Design review of the part built by this model. Coordinates are the model's own, in mm. A direction names the side the tool comes from. Coordinates: 2 decimals unless noted, no trailing zeros. Order: outer loops, then holes, each group sorted by start corner. A loop starts at its lowest first (then second) coordinate and runs counter-clockwise, first axis right, second up. Notation, with made-up numbers: M 17,72 L 55,72 A17 ccw 55,82 Z; hole C 4,35.5 d10. An arc over 180 degrees is marked long. Answer in a Markdown table with one row per item.
from build123d import *

# Parameters (mm, degrees)
BOSS_EXTRUDE1_DEPTH = 40
CUT_EXTRUDE1_DEPTH  = 10


with BuildPart() as part:
    # Sketch1 → Boss-Extrude1 (new body)
    with BuildSketch(Plane.XY):
        Polygon((0, 0), (-7.54, -7.54), (-34.44, -7.54), (-34.44, -2.54), (-9.611067812, -2.54), (0, 7.071067812), (9.611067812, -2.54), (34.44, -2.54), (34.44, -7.54), (7.54, -7.54), align=None)
    extrude(amount=BOSS_EXTRUDE1_DEPTH)

    # Sketch3 → Cut-Extrude1 (cut)
    with BuildSketch(Plane(origin=(0, -2.54, 0), x_dir=(1, 0, 0), z_dir=(0, 1, 0))):
        with BuildLine():
            Line((-24.440315349, -31.5), (-24.440315349, -37.5))
            ThreePointArc((-24.440315349, -37.5), (-22.94, -39.000315349), (-21.439684651, -37.5))
            Line((-21.439684651, -37.5), (-21.439684651, -31.5))
            ThreePointArc((-21.439684651, -31.5), (-22.94, -29.999684651), (-24.440315349, -31.5))
        make_face()
        with BuildLine():
            Line((21.439684651, -2.5), (21.439684651, -8.5))
            ThreePointArc((21.439684651, -8.5), (22.94, -10.000315349), (24.440315349, -8.5))
            Line((24.440315349, -8.5), (24.440315349, -2.5))
            ThreePointArc((24.440315349, -2.5), (22.94, -0.999684651), (21.439684651, -2.5))
        make_face()
        with BuildLine():
            Line((-24.440315349, -2.5), (-24.440315349, -8.5))
            ThreePointArc((-24.440315349, -8.5), (-22.94, -10.000315349), (-21.439684651, -8.5))
            Line((-21.439684651, -8.5), (-21.439684651, -2.5))
            ThreePointArc((-21.439684651, -2.5), (-22.94, -0.999684651), (-24.440315349, -2.5))
        make_face()
        with BuildLine():
            Line((21.439684651, -31.5), (21.439684651, -37.5))
            ThreePointArc((21.439684651, -37.5), (22.94, -39.000315349), (24.440315349, -37.5))
            Line((24.440315349, -37.5), (24.440315349, -31.5))
            ThreePointArc((24.440315349, -31.5), (22.94, -29.999684651), (21.439684651, -31.5))
        make_face()
    extrude(amount=-CUT_EXTRUDE1_DEPTH, mode=Mode.SUBTRACT)


solid = part.part
(1) Add section D-D, the plane y = 2. Give the boundary of the cut face in (x, z), and give its area (3 significant figures).
Return value:
| item | result |
|---|---|
| outline | M -5.07,0 L 5.07,0 L 5.07,40 L -5.07,40 Z |
| area | 406 mm2 |
(2) Add section B-B, the plane x = 22.94. Give the boundary of the cut face in (y, z).
Return value:
| item | result |
|---|---|
| outline | M -7.54,0 L -2.54,0 L -2.54,1 L -7.54,1 Z; M -7.54,10 L -2.54,10 L -2.54,30 L -7.54,30 Z; M -7.54,39 L -2.54,39 L -2.54,40 L -7.54,40 Z |
(3) Add section A-A, the plane z = 7. Give the boundary of the cut face in (x, y), and give its area (3 significant figures).
Return value:
| item | result |
|---|---|
| outline | M -34.44,-7.54 L -24.44,-7.54 L -24.44,-2.54 L -34.44,-2.54 Z; M -21.44,-7.54 L -7.54,-7.54 L 0,0 L 7.54,-7.54 L 21.44,-7.54 L 21.44,-2.54 L 9.61,-2.54 L 0,7.07 L -9.61,-2.54 L -21.44,-2.54 Z; M 24.44,-7.54 L 34.44,-7.54 L 34.44,-2.54 L 24.44,-2.54 Z |
| area | 350 mm2 |
(4) Insertion check: pin 1 Ø1 at (y, z) = (0, 4) entering from +X; pin 2 Ø20 at (x, z) = (-28, 17) entering from +Y; pin 3 Ø6 at (x, y) = (-18, 0.5) entering from -Z; pin 4 Ø10 at (x, z) = (8.5, 11) entering from +Y. Each pin has a flat end and moves straight along its axis. Give the tip position at first contact, or say it passes through.
Return value:
| item | result |
|---|---|
| pin 1 | stops at x = 7.57 |
| pin 2 | stops at y = -2.54 |
| pin 3 | passes through |
| pin 4 | stops at y = 3.57 |
(5) Add section C-C, the plane z = 16. Give the boundary of the cut face in (x, y), and give its area (3 significant figures).
Return value:
| item | result |
|---|---|
| outline | M -34.44,-7.54 L -7.54,-7.54 L 0,0 L 7.54,-7.54 L 34.44,-7.54 L 34.44,-2.54 L 9.61,-2.54 L 0,7.07 L -9.61,-2.54 L -34.44,-2.54 Z |
| area | 380 mm2 |
(6) Draft analysis for pull direction X (two halves, no side actions). For faces 4 (the flat face through (21.44, -5, 34)), 5 (the flat face through (-34.44, -5, 20)), 6 (the flat face through (0.5, -0.1, 0)), state which applies: pulls with the +X half, pulls with the -X half, needs draft (parallel to the pull), parting line crosses it, or undercut.
Return value:
| item | result |
|---|---|
| face 4 | undercut |
| face 5 | pulls with the -X half |
| face 6 | needs draft |
(7) For line 1 along Z through (x, y) = (-23.5, -6.5); line 2 along Y through (x, z) = (18.5, 35); line 3 along X through (y, z) = (-6, 31), list the stretches that pass through material, from the lowest coordinate up. Write a range as from..to.
Return value:
| item | result |
|---|---|
| line 1 | z = 0..1.11, 9.89..30.11, 38.89..40 |
| line 2 | y = -7.54..-2.54 |
| line 3 | x = -34.44..-24.35, -21.53..-6, 6..21.53, 24.35..34.44 |
(8) For faces 1 (the flat face through (-24.44, -5, 5)), 2 (the flat face through (4, -4, 20)), 3 (the flat face through (4.74, 2.33, 19.72)), list the 3-axis set-ups (+Z, -Z, +X, -X, +Y, -Y) from which the entire face can be reached by the end or side of a thin tool; tool diameter is ignored.
Return value:
| item | result |
|---|---|
| face 1 | +Y, -Y |
| face 2 | +Z, -Z, -Y |
| face 3 | +Z, -Z, +X, +Y |
